Geometry: see drawing. Coordinates: mm, zero at the bounding-box minimum. A direction names the side the tool comes from. Coordinates: 2 decimals unless noted, no trailing zeros. Order: outer loops, then holes, each group sorted by start corner. A loop starts at its lowest first (then second) coordinate and runs counter-clockwise, first axis right, second up. Notation, with made-up numbers: M -2,1.5 L 17,1.5 A26 ccw 17,37.5 Z; hole C 14,62.5 d7. An arc over 180 degrees is marked long. One line per item, written item: value.
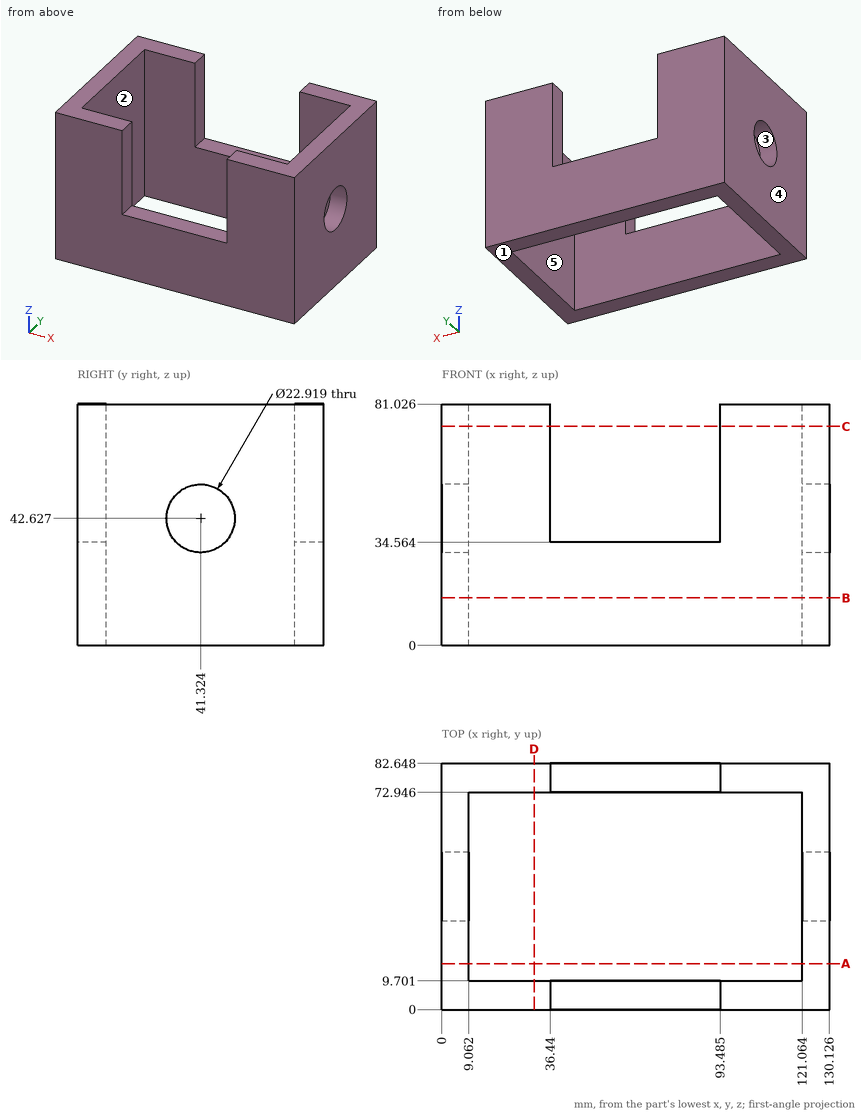
(1) Cut plane D-D on x = 31. Output: boundary loops of the cut face in (y, z).
Data:
outline: M 0,0 L 9.7,0 L 9.7,81.03 L 0,81.03 Z; M 72.95,0 L 82.65,0 L 82.65,81.03 L 72.95,81.03 Z
(2) Draft query along X for the marked faces 3, 4 and 5. Return one class per face: released by +X, released by -X, zero draft, split by the parting line, or undercut.
Data:
face 3: zero draft
face 4: released by -X
face 5: undercut
(3) Ray query, line 1 (Y direction, x = 19.5, z = 44); line 2 (X direction, y = 72, z = 47.5) (1 decimal); line 3 (Z direction, x = 49, y = 9.5). Return the intervals inside material, ascending. Write a range as from..to.
Data:
line 1: y = 0..9.7, 72.95..82.65
line 2: x = 0..9.1, 121.1..130.1
line 3: z = 0..34.56
(4) First-contact query: pin 1 (5 mm diameter, centred on x = 82.5, y = 68.5, fed in from +Z); pin 2 (5 mm diameter, centred on x = 79, y = 79.5, fed in from +Z). Flat tips, straight axial feed; report the tip coordinate or a pass-through.
Data:
pin 1: passes through
pin 2: stops at z = 34.56
(5) Access query for the marked faces 1 and 2. Directions: +Z, -Z, +X, -X, +Y, -Y. A direction counts if a zero-diameter tool reaches every point of the face in a straight line with its end or side. Return the directions, or none.
Data:
face 1: -Z, +X, -X, +Y, -Y
face 2: +Z, -Z
(6) Cut plane A-A on y = 15.5. Output: boundary loops of the cut face in (x, z) (1 decimal), plus the area to 3 significant figures.
Data:
outline: M 0,0 L 9.1,0 L 9.1,81 L 0,81 Z; M 121.1,0 L 130.1,0 L 130.1,81 L 121.1,81 Z
area: 1,470 mm2
(7) Cut plane B-B on z = 16. Output: boundary loops of the cut face in (x, y) (1 decimal), plus the area to 3 significant figures.
Data:
outline: M 0,0 L 130.1,0 L 130.1,82.6 L 0,82.6 Z; hole M 9.1,9.7 L 121.1,9.7 L 121.1,72.9 L 9.1,72.9 Z
area: 3,670 mm2
(8) Cut plane C-C on z = 73.5. Output: boundary loops of the cut face in (x, y) (1 decimal).
Data:
outline: M 0,0 L 36.4,0 L 36.4,9.7 L 9.1,9.7 L 9.1,72.9 L 36.4,72.9 L 36.4,82.6 L 0,82.6 Z; M 93.5,0 L 130.1,0 L 130.1,82.6 L 93.5,82.6 L 93.5,72.9 L 121.1,72.9 L 121.1,9.7 L 93.5,9.7 Z
